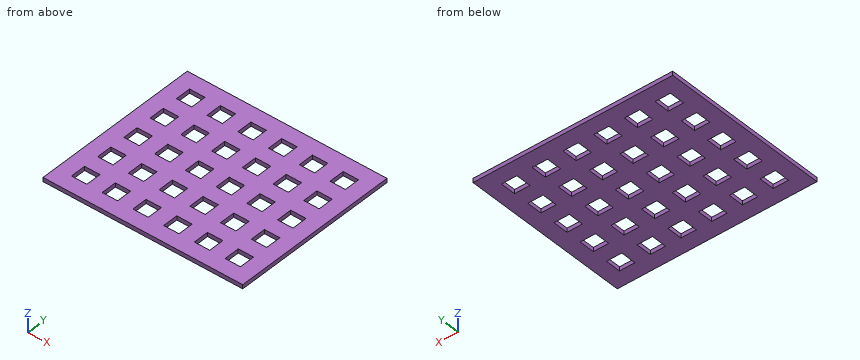
```python
from build123d import *

# Parameters (mm, degrees)
SKETCH_1_W             = 18
SKETCH_1_H             = 1.5
EXTRUDE_1_DEPTH        = 0.4
PATTERN_LINEAR_1_COUNT = 6
PATTERN_LINEAR_1_PITCH = 3
EXTRUDE_3_DEPTH        = 0.4
PATTERN_LINEAR_2_COUNT = 7
PATTERN_LINEAR_2_PITCH = 3


with BuildPart() as part:
    # Sketch 1 → Extrude 1 (new body)
    with BuildSketch(Plane.XY):
        with Locations((9, 0.75)):
            Rectangle(SKETCH_1_W, SKETCH_1_H)
    extrude(amount=EXTRUDE_1_DEPTH)


with BuildPart() as pattern_linear_1_1:
    # Pattern Linear 1: pattern copy
    add(part.part.moved(Location(Vector(0, 1, 0) * (1 * PATTERN_LINEAR_1_PITCH))))


with BuildPart() as pattern_linear_1_2:
    # Pattern Linear 1: pattern copy
    add(part.part.moved(Location(Vector(0, 1, 0) * (2 * PATTERN_LINEAR_1_PITCH))))


with BuildPart() as pattern_linear_1_3:
    # Pattern Linear 1: pattern copy
    add(part.part.moved(Location(Vector(0, 1, 0) * (3 * PATTERN_LINEAR_1_PITCH))))


with BuildPart() as pattern_linear_1_4:
    # Pattern Linear 1: pattern copy
    add(part.part.moved(Location(Vector(0, 1, 0) * (4 * PATTERN_LINEAR_1_PITCH))))


with BuildPart() as pattern_linear_1_5:
    # Pattern Linear 1: pattern copy
    add(part.part.moved(Location(Vector(0, 1, 0) * (5 * PATTERN_LINEAR_1_PITCH))))


with BuildPart() as part_1:
    add(part.part)

    add(pattern_linear_1_1.part)  # Extrude 3 merges Pattern Linear 1_1

    add(pattern_linear_1_2.part)  # Extrude 3 merges Pattern Linear 1_2

    add(pattern_linear_1_3.part)  # Extrude 3 merges Pattern Linear 1_3
    # Sketch 3 → Extrude 3 (add)
    with BuildSketch(Plane.XY.offset(0.4)):
        Polygon((0, 16.5), (0, 10.5), (0, 0), (-1.5, 0), (-1.5, 10.98507125), (-1.5, 16.5), align=None)
    extrude_3 = extrude(amount=-EXTRUDE_3_DEPTH)

    # Pattern Linear 2: Extrude 3 ×7
    with Locations(*[(i * PATTERN_LINEAR_2_PITCH, 0, 0) for i in range(1, PATTERN_LINEAR_2_COUNT)]):
        add(extrude_3)

    # Combine 1: read off the stored shape, not the designer's step
    # Combine 1: union Pattern Linear 1_4, Pattern Linear 1_5
    add(pattern_linear_1_4.part)
    add(pattern_linear_1_5.part)


solid = part_1.part
```
The listing builds one solid part. Answer for the finished solid, in the listing's coordinates (mm). Coordinates: 2 decimals unless noted, no trailing zeros. Loops run counter-clockwise (first coordinate to the right, second up) from the corner with the lowest first, then second, coordinate; pieces in that order, holes last. Notation, with made-up numbers: M 59,-15 L 116,-15 A14 ccw 116,-6 Z; hole C 46.5,47.25 d11. An arc over 180 degrees is marked long. Answer as a JSON object with one key per item and string values. Group by question number.
Item 1: Section A-A (x = 4.25) is taken. Write down the section's boundary in (y, z).
Item 2: Section B-B (y = 5.25) is taken. Write down the section's boundary in (x, z).
Item 3: Consider L1, parallel to Y at x = 7, z = 0.1. Determine where the line is inside the solid, lowest interval first.
Item 4: Section C-C (z = 0.3) is taken. Give the number of separate pieces and of enclosed holes in the cut face, and give its area (3 significant figures).
Solved:
{
 "1": {"outline": "M 0,0 L 1.5,0 L 1.5,0.4 L 0,0.4 Z; M 3,0 L 4.5,0 L 4.5,0.4 L 3,0.4 Z; M 6,0 L 7.5,0 L 7.5,0.4 L 6,0.4 Z; M 9,0 L 10.5,0 L 10.5,0.4 L 9,0.4 Z; M 12,0 L 13.5,0 L 13.5,0.4 L 12,0.4 Z; M 15,0 L 16.5,0 L 16.5,0.4 L 15,0.4 Z"},
 "2": {"outline": "M -1.5,0 L 0,0 L 0,0.4 L -1.5,0.4 Z; M 1.5,0 L 3,0 L 3,0.4 L 1.5,0.4 Z; M 4.5,0 L 6,0 L 6,0.4 L 4.5,0.4 Z; M 7.5,0 L 9,0 L 9,0.4 L 7.5,0.4 Z; M 10.5,0 L 12,0 L 12,0.4 L 10.5,0.4 Z; M 13.5,0 L 15,0 L 15,0.4 L 13.5,0.4 Z; M 16.5,0 L 18,0 L 18,0.4 L 16.5,0.4 Z"},
 "3": {"L1": "y = 0 to 1.5, 3 to 4.5, 6 to 7.5, 9 to 10.5, 12 to 13.5, 15 to 16.5"},
 "4": {"separate pieces": "1", "enclosed holes": "30", "area": "254 mm2"}
}
